from build123d import *

# Parameters (mm, degrees)
SKETCH2_W           = 80
SKETCH2_H           = 60
BOSS_EXTRUDE2_DEPTH = 50
CUT_EXTRUDE1_DEPTH  = 51
CUT_EXTRUDE3_DEPTH  = 51
SKETCH10_R          = 5
CUT_EXTRUDE4_DEPTH  = 58.795911827


with BuildPart() as part:
    # Sketch2 → Boss-Extrude2 (new body)
    with BuildSketch(Plane(origin=(0, 0, 0), x_dir=(1, 0, 0), z_dir=(0, 1, 0))):
        Rectangle(SKETCH2_W, SKETCH2_H)
    extrude(amount=BOSS_EXTRUDE2_DEPTH)

    # Sketch4 → Cut-Extrude1 (cut, through all)
    with BuildSketch(Plane(origin=(0, 50, 0), x_dir=(1, 0, 0), z_dir=(0, 1, 0))):
        Polygon((0, -30), (40, 30), (40, -30), align=None)
    extrude(amount=-CUT_EXTRUDE1_DEPTH, mode=Mode.SUBTRACT)

    # Sketch9 → Cut-Extrude3 (cut, through all)
    with BuildSketch(Plane(origin=(0, 50, 0), x_dir=(1, 0, 0), z_dir=(0, 1, 0))):
        Polygon((23.307672553, 4.96150883), (21.177929754, 17.573832829), (-3.871292132, -20), (6.666666667, -20), align=None)
    extrude(amount=-CUT_EXTRUDE3_DEPTH, mode=Mode.SUBTRACT)

    # Sketch10 → Cut-Extrude4 (cut, through all)
    with BuildSketch(Plane(origin=(6.550643909, 0, 4.367095939), x_dir=(0.554700196, 0, -0.832050294), z_dir=(0.832050294, 0, 0.554700196))):
        with Locations((3.790651088, 27.7575331)):
            Circle(SKETCH10_R)
    extrude(amount=-CUT_EXTRUDE4_DEPTH, mode=Mode.SUBTRACT)


solid = part.part
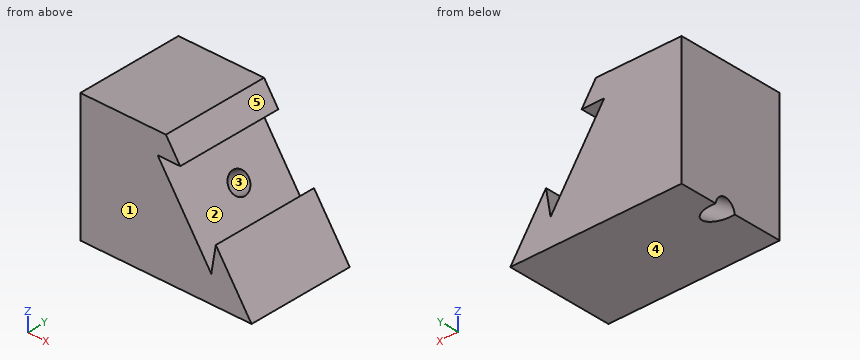
Check sheet for the modelled part. Datum: model origin and axes. Units: mm. Face numbers are marked on the shaded views. A direction names the side the tool comes from. Give positions to 0.01 mm unless a question says otherwise; leave off trailing zeros. Write each loop counter-clockwise with the first axis right and the second up, starting at its lowest first coordinate (ties: lowest second). Pieces come first, ordered by that corner, then holes. Notation, with made-up numbers: M 66,33.5 L 91,33.5 A17 cw 91,66.5 Z; hole C 7.5,46 d3. An arc over 180 degrees is marked long. Use one line per item in the form item = value.
(1) Draft check along Z on the marked faces 3, 4 and 5. Enter one of: pulls with the +Z half, pulls with the -Z half, needs draft (parallel to the pull), parting line crosses it, or undercut.
Answer block:
face_3 = undercut
face_4 = pulls with the -Z half
face_5 = pulls with the +Z half
(2) Depth check by flat-ended pin: P1, Ø8, axis at y = 7, z = -6, coming from the +X side; P2, Ø12, axis at x = 18, z = 0.5, coming from the -Y side; P3, Ø5, axis at x = -23, z = 11, coming from the -Y side; P4, Ø12, axis at x = 11.5, y = 22.5, coming from the +Z side. Enter the tip coordinate at first touch or a pass-through.
Answer block:
P1 = 26.67
P2 = through
P3 = 0
P4 = 21.75
(3) Section check A-A on y = 17.5. Record the boundary of the cut face in (x, z), plus the area to 3 significant figures.
Answer block:
outline = M -40,-30 L 40,-30 L 23.31,-4.96 L 21.18,-17.57 L -3.87,20 L 6.67,20 L 0,30 L -40,30 Z
area = 3,270 mm2
(4) Section check B-B on z = -9. State how many separate pieces and enclosed holes the cut face has, plus the area to 3 significant figures.
Answer block:
separate_pieces = 2
enclosed_holes = 1
area = 2,800 mm2
(5) Material ranges on line 1 along Y through (x, z) = (8, 0.5); line 2 along X through (y, z) = (17, -13.5); line 3 along Y through (x, z) = (-20.5, -14.5), recorded low to high.
Answer block:
line_1 = 0 to 22.76, 32.75 to 50
line_2 = -40 to 18.46, 21.87 to 29
line_3 = 0 to 23.83, 31.68 to 50
(6) Tool access check on the marked faces 1 and 2. Record the directions out of +Z, -Z, +X, -X, +Y, -Y that give a thin tool (end or side, any length) a straight path to the whole face; none if there is none.
Answer block:
face_1 = +Z, -Z, +X, -X, -Y
face_2 = +Y, -Y
(7) Section check C-C on x = 29. Record the boundary of the cut face in (y, z), plus the area to 3 significant figures.
Answer block:
outline = M 0,-30 L 50,-30 L 50,-13.5 L 0,-13.5 Z
area = 825 mm2
